Autodesk Inventor part; units mm, degrees
ref_plane "YZ Plane" through (0, 0, 0) normal (1, 0, 0) x (0, 1, 0)
ref_plane "XZ Plane" through (0, 0, 0) normal (0, 1, 0) x (-1, 0, 0)
ref_plane "XY Plane" through (0, 0, 0) normal (0, 0, 1) x (1, 0, 0)
sketch "Esboço1" plane through (0, 0, 0) normal (0, 0, 1) x (1, 0, 0)
  line L0 (-3, 2) -> (3, 2)
  line L1 (3, 2) -> (3, -2)
  line L2 (3, -2) -> (-3, -2)
  line L3 (-3, -2) -> (-3, 2)
  line L4 (-3, 2) -> (3, -2) construction
  line L5 (3, 2) -> (-3, -2) construction
  point P0 (0, 0)
  dimension "d0" = 6
  dimension "d1" = 4
extrude "Extrusão1" add sketch "Esboço1" along normal blind 24
chamfer "Chanfro1" distance 3 angle 45 2 edges at (3, 0, 24) (-3, 0, 24)
properties part number "PEÇA MOVEL"
Read the model definition and answer for the solid it produces. Units are mm, in the model's axes. Round coordinates to 2 decimals unless told otherwise and drop trailing zeros. Order: outer loops, then holes, each group sorted by start corner. A loop starts at its lowest first (then second) coordinate and runs counter-clockwise, first axis right, second up.
1) The part is cut by section B-B on x = 0.75. Write down the section's boundary in (y, z).
2) The part is cut by section C-C on x = 2.5. Write down the section's boundary in (y, z).
3) A flat-ended cylindrical pin translates along its axis: pin 1 (2 mm diameter, centred on x = 2, y = 1.5, fed in from +Z). Find the tip coordinate at first contact, or state that the pin passes through.
4) Straight lines are drawn through the part: L1, parallel to Z at x = -0.5, y = -1.5; L2, parallel to Z at x = 2.5, y = 0.45; L3, parallel to X at y = -0.6, z = 21.5. For each, find the intervals that lie inside material, in ascending order.
Resolved:
1. outline: (-2, 0) - (2, 0) - (2, 23.25) - (-2, 23.25) - close
2. outline: (-2, 0) - (2, 0) - (2, 21.5) - (-2, 21.5) - close
3. pin 1: stops at z = 23
4. L1: z = 0 to 23.5
4. L2: z = 0 to 21.5
4. L3: x = -2.5 to 2.5
